Autodesk Inventor part; units mm, degrees
ref_plane "YZ Plane" through (0, 0, 0) normal (1, 0, 0) x (0, 1, 0)
ref_plane "XZ Plane" through (0, 0, 0) normal (0, 1, 0) x (-1, 0, 0)
ref_plane "XY Plane" through (0, 0, 0) normal (0, 0, 1) x (1, 0, 0)
sketch "Sketch1" plane through (0, 0, 0) normal (0, 0, 1) x (1, 0, 0)
  circle A0 centre (0, 0) radius 15.5
  dimension "d0" = 31
extrude "Extrusion1" add sketch "Sketch1" along normal blind 30
sketch "Sketch2" plane through (0, 0, 30) normal (0, 0, 1) x (1, 0, 0)
  circle A0 centre (0, 0) radius 18.4
  dimension "d3" = 36.8
extrude "Extrusion2" add sketch "Sketch2" along normal blind 24
sketch "Sketch3" plane through (0, 0, 54) normal (0, 0, 1) x (1, 0, 0)
  line L0 (0, 0) -> (7, 0)
  circle A0 centre (7, 0) radius 3
  circle A1 centre (7, 0) radius 6
  dimension "d6" = 7
  dimension "d7" = 6
  dimension "d8" = 12
extrude "Extrusion3" add sketch "Sketch3" along normal blind 22 contours A0
extrude "Extrusion4" add sketch "Sketch3" along normal blind 6.5
chamfer "Chamfer1" distance 1 angle 45 1 edges at (1, 0, 60.5)
sketch "Sketch4" plane through (7, 0, 76) normal (0, 0, 1) x (1, 0, 0)
  point P0 (-7, 0)
sketch "Sketch5" plane through (7, 0, 76) normal (0, 0, 1) x (1, 0, 0)
  line L0 (0, 0) -> (-2.4, 0)
  line L1 (-2.4, 0) -> (-2.4, -1.7999)
  line L2 (-2.4, 0) -> (-2.4, 1.8068)
  arc A0 (-2.4, 1.8068) -> (-2.4, -1.7999) centre (-0.0145, 0.0034) ccw
  point P0 (-7, 0)
  dimension "d16" = 2.4
extrude "Extrusion5" cut sketch "Sketch5" against normal blind 12
sketch "Sketch6" plane through (4.6, -1.7999, 76) normal (-1, 0, 0) x (0, 0, 1)
  line L0 (-11.9968, 1.7999) -> (-7.9968, 1.7999)
  circle A0 centre (-7.9968, 1.7999) radius 0.5
  point P0 (-76, 1.7999)
  dimension "d19" = 4
  dimension "d20" = 1
sketch "Sketch8" plane through (0, 0, 54) normal (0, 0, 1) x (1, 0, 0)
  point P0 (0, 0)
sketch "Sketch9" plane through (0, 0, 54) normal (0, 0, 1) x (1, 0, 0)
  line L0 (0, 0) -> (0, 16.95)
  circle A0 centre (0, 16.95) radius 1.25
  line L1 (0, 0) -> (0, -16.95)
  circle A1 centre (0, -16.95) radius 1.25
  line L2 (0, 0) -> (-16.95, 0)
  circle A2 centre (-16.95, 0) radius 1.25
  line L3 (0, -16.95) -> (-13.7744, -9.8425)
  circle A3 centre (-13.7744, -9.8425) radius 1.25
  circle A4 centre (-13.7744, 9.8425) radius 1.25
  line L4 (0, 16.95) -> (-13.7744, 9.8425)
  line L5 (-13.7744, -9.8425) -> (-13.7744, 9.8425)
  line L6 (0, -16.95) -> (13.7744, -9.8425)
  circle A5 centre (13.7744, -9.8425) radius 1.25
  line L7 (0, 16.95) -> (13.7744, 9.8425)
  circle A6 centre (13.7744, 9.8425) radius 1.25
  line L8 (0, 0) -> (13.7744, 0)
  line L9 (13.7744, 0) -> (13.7744, -9.8425)
  dimension "d49" = 16.95
  dimension "d50" = 2.5
  dimension "d51" = 16.95
  dimension "d52" = 2.5
  dimension "d66" = 16.95
  dimension "d67" = 2.5
  dimension "d68" = 15.5
  dimension "d69" = 2.5
  dimension "d71" = 2.5
  dimension "d72" = 15.5
  dimension "d116" = 2.5
  dimension "d117" = 2.5
hole "Hole2" at (0, -16.95, 54) direction (0, 0, -1) diameter 2.5 end through all
extrude "Extrusion9" cut sketch "Sketch9" against normal through all contours A0 L4 L0 | L0 L7 A0 | L4 A0 L7
thread "Thread5"
thread "Thread6"
hole "Hole3" at (-13.7744, -9.8425, 54) direction (0, 0, -1) diameter 2.5 end through all
hole "Hole4" at (-13.7744, 9.8425, 54) direction (0, 0, -1) diameter 2.5 end through all
thread "Thread7"
thread "Thread8"
hole "Hole7" at (-16.95, 0, 54) direction (0, 0, -1) diameter 2.5 end through all
thread "Thread9"
hole "Hole8" at (13.7744, -9.8425, 54) direction (0, 0, -1) diameter 2.5 end through all
hole "Hole9" at (13.7744, 9.8425, 54) direction (0, 0, -1) diameter 2.5 end through all
thread "Thread10"
thread "Thread11"
thread "Thread12"
equation "\"d58\" = Thickness"
equation "\"d78\" = Thickness"
equation "\"d85\" = Thickness"
equation "\"d110\" = Thickness"
equation "\"d123\" = Thickness"
equation "\"d130\" = Thickness"
equation "\"BendRadius\" = Thickness"
equation "\"BendReliefWidth\" = Thickness"
equation "\"BendReliefDepth\" = 0.5 * Thickness"
equation "\"CornerReliefSize\" = 4 * Thickness"
equation "\"MinimumRemnant\" = 2 * Thickness"
equation "\"TransitionRadius\" = BendRadius"
equation "\"JacobiRadiusSize\" = BendRadius"
equation "\"GapSize\" = Thickness"
properties part number "motor_polulu"
The model under review builds one solid part; all positions refer to its coordinate system, in mm. A direction names the side the tool comes from. Coordinates: 2 decimals unless noted, no trailing zeros. Write each loop counter-clockwise with the first axis right and the second up, starting at its lowest first coordinate (ties: lowest second). Pieces come first, ordered by that corner, then holes. Notation, with made-up numbers: (-32, 36) -> (16, 36) arc R20 ccw to (16, 55) -> close; hole circle Ø8 at (-35.5, 25). An arc over 180 degrees is marked (long way). Answer in a Markdown table with one row per item.
1. Clearance check with flat-ended pins moving along their axes: pin 1 Ø5 at (x, z) = (5.5, 54.5) entering from +Y; pin 2 Ø10 at (y, z) = (4.5, 27.5) entering from +X; pin 3 Ø1.1 at (y, z) = (0, 71) entering from -X. State where each tip first meets the part, or that it passes through.
Answers below:
| item | result |
|---|---|
| pin 1 | stops at y = 18.15 |
| pin 2 | stops at x = 18.4 |
| pin 3 | stops at x = 4.6 |
2. Wall thickness on probe 1 along Y at (x, z) = (0, 41); probe 2 along Y at (x, z) = (1, 34.5); probe 3 along Y at (x, z) = (-16.95, 35.75): over which ranges is each line inside the solid? List them lowest first. Write a range as [from, to].
Answers below:
| item | result |
|---|---|
| probe 1 | y = [-18.4, -18.2], [-15.7, 15.7], [18.2, 18.4] |
| probe 2 | y = [-18.37, -17.7], [-16.2, 16.2], [17.7, 18.37] |
| probe 3 | y = [-7.16, -1.25], [1.25, 7.16] |
3. We need section A-A, the plane y = 0. State the section outline as (x, z) points.
Answers below:
| item | result |
|---|---|
| outline | (-18.4, 30) -> (-18.2, 30) -> (-18.2, 54) -> (-18.4, 54) -> close; (-15.7, 30) -> (-15.5, 30) -> (-15.5, 0) -> (15.5, 0) -> (15.5, 30) -> (18.4, 30) -> (18.4, 54) -> (13, 54) -> (13, 59.5) -> (12, 60.5) -> (10, 60.5) -> (10, 76) -> (4.6, 76) -> (4.6, 64) -> (4, 64) -> (4, 60.5) -> (2, 60.5) -> (1, 59.5) -> (1, 54) -> (-15.7, 54) -> close |
4. We need section B-B, the plane x = 0. State the section outline as (y, z) points.
Answers below:
| item | result |
|---|---|
| outline | (-18.4, 30) -> (-18.2, 30) -> (-18.2, 54) -> (-18.4, 54) -> close; (-15.7, 30) -> (-15.5, 30) -> (-15.5, 0) -> (15.5, 0) -> (15.5, 30) -> (15.7, 30) -> (15.7, 54) -> (-15.7, 54) -> close; (18.2, 30) -> (18.4, 30) -> (18.4, 54) -> (18.2, 54) -> close |
5. We need section C-C, the plane y = -10. State the section outline as (x, z) points, and give its area (3 significant figures).
Answers below:
| item | result |
|---|---|
| outline | (-15.45, 30) -> (-15.01, 30) -> (-15.01, 54) -> (-15.45, 54) -> close; (-12.53, 30) -> (-11.84, 30) -> (-11.84, 0) -> (11.84, 0) -> (11.84, 30) -> (12.53, 30) -> (12.53, 54) -> (-12.53, 54) -> close; (15.01, 30) -> (15.45, 30) -> (15.45, 54) -> (15.01, 54) -> close |
| area | 1,330 mm^2 |
6. We need section D-D, the plane x = -16.95. State the section outline as (y, z) points, and give its area (3 significant figures).
Answers below:
| item | result |
|---|---|
| outline | (-7.16, 30) -> (-1.25, 30) -> (-1.25, 54) -> (-7.16, 54) -> close; (1.25, 30) -> (7.16, 30) -> (7.16, 54) -> (1.25, 54) -> close |
| area | 284 mm^2 |
7. For faces 1 (the cylindrical face through (-12.554, -9.572, 41.832)), 2 (the flat face through (4.6, 0, 70)), 3 (the cylindrical face through (-2.018, -15.368, 14.79)), 4 (the cylindrical face through (1, 0, 57)), 5 (the flat face through (0, 0, 0)), list the 3-axis set-ups (+Z, -Z, +X, -X, +Y, -Y) from which the entire face can be reached by the end or side of a thin tool; tool diameter is ignored.
Answers below:
| item | result |
|---|---|
| face 1 | +Z, -Z |
| face 2 | +Z, -X, +Y, -Y |
| face 3 | -Z |
| face 4 | +Z |
| face 5 | -Z, +X, -X, +Y, -Y |
8. Draft analysis for pull direction X (two halves, no side actions). For faces 6 (the cylindrical face through (-18.004, -0.672, 41.832)), 7 (the cylindrical face through (9.77, 1.15, 68.14)), 8 (the flat face through (10.3, 0.1, 60.5)), state which applies: +X half, -X half, draft (parallel to the pull), parting line (faces both ways), or undercut.
Answers below:
| item | result |
|---|---|
| face 6 | undercut |
| face 7 | parting line |
| face 8 | draft |
